from build123d import *

# Parameters (mm, degrees)
F0_W     = 40
F0_H     = 10
F1_DEPTH = 4
F2_W     = 16
F2_H     = 1.5
F3_DEPTH = 8
F4_W     = 8
F4_H     = 5.5
F5_DEPTH = 6
F6_R     = 1
F7_SIZE  = 6


# Not quite as in the source:
# - a feature names something its author has since deleted; it is built from what else it names


with BuildPart() as f1:
    # F0 (on Front) → F1 (new body)
    with BuildSketch(Plane.XZ):
        Rectangle(F0_W, F0_H)
        with BuildLine():
            Line((-12.25, -1.5), (-12.25, 0.5))
            ThreePointArc((-12.25, 0.5), (-10, 2.75), (-7.75, 0.5))
            Line((-7.75, 0.5), (-7.75, -1.5))
            ThreePointArc((-7.75, -1.5), (-10, -3.75), (-12.25, -1.5))
        make_face(mode=Mode.SUBTRACT)
        with BuildLine():
            ThreePointArc((7.75, 0.5), (10, 2.75), (12.25, 0.5))
            Line((12.25, 0.5), (12.25, -1.5))
            ThreePointArc((12.25, -1.5), (10, -3.75), (7.75, -1.5))
            Line((7.75, -1.5), (7.75, 0.5))
        make_face(mode=Mode.SUBTRACT)
    extrude(amount=F1_DEPTH)

    # F2 (on face) → F3 (join)
    with BuildSketch(Plane.XZ.offset(4)):
        Polygon((4, 5), (-4, 5), (-4, 3.5), (-4, -5), (4, -5), (4, 3.5), align=None)
        with Locations((-12, 4.25)):
            Rectangle(F2_W, F2_H)
        with Locations((12, 4.25)):
            Rectangle(F2_W, F2_H)
    extrude(amount=F3_DEPTH)

    # F4 (on face) → F5 (join)
    with BuildSketch(Plane(origin=(0, 0, -5), x_dir=(1, 0, 0), z_dir=(0, 0, -1))):
        with Locations((0, 9.25)):
            Rectangle(F4_W, F4_H)
    extrude(amount=F5_DEPTH)

    # F6
    f6_edges = [f1.edges().sort_by_distance(p)[0] for p in [
        (4, -4, -0.75),
        (-4, -4, -0.75),
        (-12, -4, 3.5),
        (12, -4, 3.5),
        (4, -8, 3.5),
        (-4, -8, 3.5),
    ]]
    fillet(f6_edges, radius=F6_R)

    # F7
    f7_edges = [f1.edges().sort_by_distance(p)[0] for p in [
        (-20, -12, 4.25),
        (20, -12, 4.25),
        (20, -2, -5),
        (-20, -2, -5),
    ]]
    chamfer(f7_edges, length=F7_SIZE)


solid = f1.part
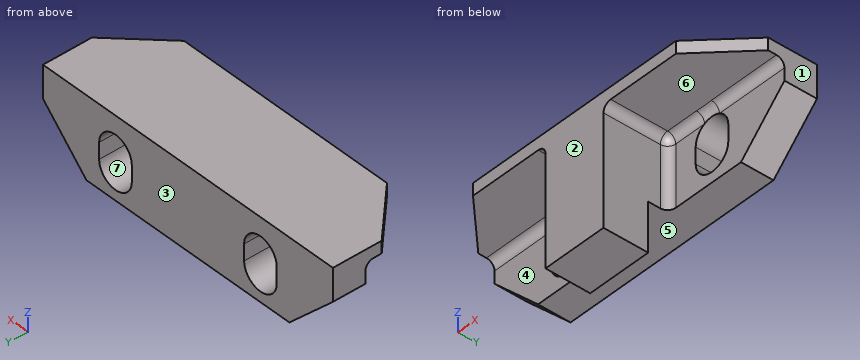
The listing builds one solid part. Answer for the finished solid, in the listing's coordinates (mm). Face numbers are marked on the shaded views. A direction names the side the tool comes from. Round coordinates to 2 decimals unless told otherwise and drop trailing zeros. Write each loop counter-clockwise with the first axis right and the second up, starting at its lowest first coordinate (ties: lowest second). Pieces come first, ordered by that corner, then holes. Notation, with made-up numbers: M 50,27 L 56,27 A16 ccw 56,43 Z; hole C 76.5,87 d10. An arc over 180 degrees is marked long. Write each question's results on one line, items separated by ' | '. Start each with the question number.
Item 1: A cutting plane is placed at C-C on y = -7.75. Write down the section's boundary in (x, z), and give its area (3 significant figures).
Item 2: For a pull along Y with two mould halves and no side action, classify the marked faces 1, 2 and 3 as pulls with the +Y half, pulls with the -Y half, needs draft (parallel to the pull), parting line crosses it, or undercut.
Item 3: A cutting plane is placed at B-B on x = -16. Write down the section's boundary in (y, z).
Item 4: For the marked faces 4, 5, 6 and 7, determine the directions among +Z, -Z, +X, -X, +Y, -Y from which every point of the face is accessible in a straight line to the end or side of a thin tool.
Item 5: A cutting plane is placed at D-D on x = 8.5. Write down the section's boundary in (y, z).
Item 6: A cutting plane is placed at A-A on y = -2.75. Write down the section's boundary in (x, z), and give its area (3 significant figures).
Item 7: Flat-ended cylindrical pins translate along their axes: pin 1 Ø1.5 at (x, z) = (13, -2.5) entering from -Y; pin 2 Ø1 at (y, z) = (-2, 0) entering from +X; pin 3 Ø1 at (y, z) = (-1, -0.5) entering from +X; pin 4 Ø8 at (x, z) = (13, 0) entering from -Y. Find the tip coordinate at first contact, or state that the pin passes through.
Item 8: Straight lines are drawn through the part: L1, parallel to X at y = -2.5, z = -1.5; L2, parallel to X at y = -8, z = -8; L3, parallel to Z at x = -7, y = -10.75. For each, find the intervals that lie inside material, in ascending order. Write a range as [from, to].
Check sheet entries:
1) outline: M -18.25,3.5 L -5,3.5 A1 cw -4,2.5 L -4,-11 L 4,-11 L 4,2.5 A1 cw 5,3.5 L 18.25,3.5 L 18.25,5 L -18.25,5 Z | area: 171 mm²
2) face 1: needs draft | face 2: pulls with the -Y half | face 3: pulls with the +Y half
3) outline: M -10,3.5 L -5,3.5 A1 cw -4,2.5 L -4,-3 L 0,-3 L 0,5 L -10,5 Z
4) face 4: -Z, -X, -Y | face 5: -Z, +X, -X, +Y | face 6: -Z, +X, -Y | face 7: +Y, -Y
5) outline: M -12,3.5 L -5,3.5 A1 cw -4,2.5 L -4,2.18 L 0,2.18 L 0,5 L -12,5 Z; M -4,-5 L 0,-5 L 0,-3.18 L -4,-3.18 Z
6) outline: M -20,1 L -14,-5 L 14,-5 L 20,1 L 20,5 L -20,5 Z; hole M -12.25,-1.5 A2.25 ccw -7.75,-1.5 L -7.75,0.5 A2.25 ccw -12.25,0.5 Z; hole M 7.75,-1.5 A2.25 ccw 12.25,-1.5 L 12.25,0.5 A2.25 ccw 7.75,0.5 Z | area: 314 mm²
7) pin 1: y = -4 | pin 2: x = 19.5 | pin 3: x = 19 | pin 4: y = -12
8) L1: [-17.5, -12.25], [-7.75, 7.75], [12.25, 17.5] | L2: [-4, 4] | L3: [3.5, 5]
